Could you check a few things on this model? Use its own coordinates, in mm. Face numbers are marked on the shaded views. Give positions to 0.01 mm unless a question says otherwise; leave off trailing zeros. Write each loop counter-clockwise with the first axis right and the second up, starting at its lowest first coordinate (ties: lowest second). Pieces come first, ordered by that corner, then holes. Notation, with made-up numbers: (45.5, 77.25) - (96.5, 77.25) arc R5 ccw to (96.5, 85.25) - close; hole circle Ø6 at (67.25, 9). An arc over 180 degrees is marked (long way). Answer as a JSON object with one key per item and string values. Group by question number.
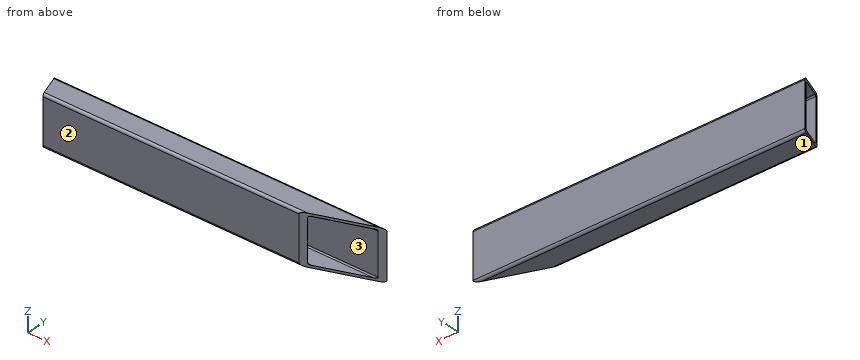
```python
from build123d import *

# Parameters (mm, degrees)
F0_W     = 344.4875
F0_H     = 50.8
F1_DEPTH = 12.7
F2_T     = -2.54
F4_DEPTH = 50.801
F6_DEPTH = 50.801
F7_R     = 2.54
F8_R     = 1.27


# Not quite as in the source:
# - a feature names something its author has since deleted; it is built from what else it names


with BuildPart() as f1:
    # F0 (on Front) → F1 (new body, symmetric)
    with BuildSketch(Plane.XZ):
        Rectangle(F0_W, F0_H)
    extrude(amount=F1_DEPTH, both=True)

    # F2
    f2_openings = [f1.faces().sort_by_distance(p)[0] for p in [
        (-172.24375, 0, 0),
        (172.24375, 0, 0),
    ]]
    offset(amount=F2_T, openings=f2_openings)

    # F3 (on face) → F4 (cut, through all)
    with BuildSketch(Plane.XY.offset(25.4)):
        Polygon((-162.9989060496, -12.7), (-172.24375, 12.7), (-172.24375, -12.7), align=None)
    extrude(amount=-F4_DEPTH, mode=Mode.SUBTRACT)

    # F5 (on face) → F6 (cut, through all)
    with BuildSketch(Plane.XY.offset(25.4)):
        Polygon((172.24375, -12.7), (172.24375, 12.7), (102.4578235459, -12.7), align=None)
    extrude(amount=-F6_DEPTH, mode=Mode.SUBTRACT)

    # F7
    f7_edges = [f1.edges().sort_by_distance(p)[0] for p in [
        (-30.270541, -12.7, 25.4),
        (0, 12.7, 25.4),
        (0, 12.7, -25.4),
        (-30.270541, -12.7, -25.4),
    ]]
    fillet(f7_edges, radius=F7_R)

    # F8
    f8_edges = [f1.edges().sort_by_distance(p)[0] for p in [
        (-27.243487, -10.16, -22.86),
        (-27.243487, -10.16, 22.86),
        (-3.027054, 10.16, 22.86),
        (-3.027054, 10.16, -22.86),
    ]]
    fillet(f8_edges, radius=F8_R)


solid = f1.part
```
(1) I want a section at D-D, the plane x = 124.5. Please give me the cut outline in (y, z).
(2) Will these pins go through, and if not, where does the flat tip stop? P1, Ø10, axis at y = -9, z = -20, coming from the -X side; P2, Ø3, axis at y = -4, z = -19.5, coming from the -X side.
(3) I want a section at A-A, the plane z = -1.5. Please give me the cut outline in (x, y).
(4) I want a section at B-B, the plane y = 6. Please give me the cut outline in (x, z), and give its area (3 significant figures).
(5) If we mould it in two halves opening along Y, with no side actions, what happens to the marked faces 1, 2 and 3? For each: +Y half, -Y half, draft (parallel to the pull), parting line (faces both ways), or undercut.
(6) I want a section at C-C, the plane x = 77. Please give me the cut outline in (y, z), and give its area (3 significant figures).
(7) I need wall thicknesses on L1, parallel to Y at x = 93.5, z = 9; L2, parallel to Z at x = -107, y = -8; L3, parallel to Z at x = 3.5, y = -9.25. Which ranges of each line are inside material? Lowest first, please.
Entries:
{
 "1": {"outline": "(-4.68, -25.4) - (10.16, -25.4) arc R2.54 ccw to (12.7, -22.86) - (12.7, 22.86) arc R2.54 ccw to (10.16, 25.4) - (-4.68, 25.4) - (-4.68, 22.86) - (8.89, 22.86) arc R1.27 cw to (10.16, 21.59) - (10.16, -21.59) arc R1.27 cw to (8.89, -22.86) - (-4.68, -22.86) - close"},
 "2": {"P1": "x = -165.84", "P2": "through"},
 "3": {"outline": "(-172.24, 12.7) - (-171.32, 10.16) - (165.27, 10.16) - (172.24, 12.7) - close; (-163.92, -10.16) - (-163, -12.7) - (102.46, -12.7) - (109.44, -10.16) - close"},
 "4": {"outline": "(-169.81, -25.4) - (153.84, -25.4) - (153.84, -22.86) - (-169.81, -22.86) - close; (-169.81, 22.86) - (153.84, 22.86) - (153.84, 25.4) - (-169.81, 25.4) - close", "area": "1,640 mm^2"},
 "5": {"face 1": "draft", "face 2": "-Y half", "face 3": "undercut"},
 "6": {"outline": "(-12.7, -22.86) arc R2.54 ccw to (-10.16, -25.4) - (10.16, -25.4) arc R2.54 ccw to (12.7, -22.86) - (12.7, 22.86) arc R2.54 ccw to (10.16, 25.4) - (-10.16, 25.4) arc R2.54 ccw to (-12.7, 22.86) - close; hole (-10.16, -21.59) arc R1.27 ccw to (-8.89, -22.86) - (8.89, -22.86) arc R1.27 ccw to (10.16, -21.59) - (10.16, 21.59) arc R1.27 ccw to (8.89, 22.86) - (-8.89, 22.86) arc R1.27 ccw to (-10.16, 21.59) - close", "area": "357 mm^2"},
 "7": {"L1": "-12.7 to -10.16, 10.16 to 12.7", "L2": "-25.4 to -22.86, 22.86 to 25.4", "L3": "-25.4 to -22.81, 22.81 to 25.4"}
}
